Check sheet for the modelled part. Datum: model origin and axes. Units: mm. A direction names the side the tool comes from. Round coordinates to 2 decimals unless told otherwise and drop trailing zeros. Loops run counter-clockwise (first coordinate to the right, second up) from the corner with the lowest first, then second, coordinate; pieces in that order, holes last. Notation, with made-up numbers: (54.25, -10) -> (80.25, -10) arc R20 ccw to (80.25, 6) -> close; hole circle Ø8 at (13.5, 47). An arc over 180 degrees is marked (long way). One line per question, with ' | ' between items.
```python
from build123d import *

# Parameters (mm, degrees)
SKETCH_1_R          = 2.5
EXTRUDE_1_DEPTH     = 8
CHAMFER_2_SIZE      = 0.5
SKETCH_2_R          = 3.5
EXTRUDE_2_DEPTH     = 1.5
DOME_1_FACE_RADIUS  = 3.5
DOME_1_HEIGHT       = 0.8
SKETCH_3_W          = 2.012887991
SKETCH_3_H          = 3.133753739
CUT_EXTRUDE_1_DEPTH = 5


with BuildPart() as part:
    # 草图1 → 凸台-拉伸1 (new body)
    with BuildSketch(Plane.XY):
        Circle(SKETCH_1_R)
    extrude(amount=EXTRUDE_1_DEPTH)

    # 倒角2
    chamfer_2_edges = [part.edges().sort_by_distance(p)[0] for p in [
        (-2.5, 0, 8),
    ]]
    chamfer(chamfer_2_edges, length=CHAMFER_2_SIZE)

    # 草图2 → 凸台-拉伸2 (add)
    with BuildSketch(Plane(origin=(0, 0, 0), x_dir=(-1, 0, 0), z_dir=(0, 0, -1))):
        Circle(SKETCH_2_R)
    extrude(amount=EXTRUDE_2_DEPTH)

    # 圆顶1: a dome of height H over a round flat face of radius A is a cap of a sphere of radius (A * A + H * H) / (2 * H)
    dome_1_r = (DOME_1_FACE_RADIUS * DOME_1_FACE_RADIUS + DOME_1_HEIGHT * DOME_1_HEIGHT) / (2 * DOME_1_HEIGHT)
    dome_1_base = Plane((0, 0, -1.5), z_dir=(0, 0, -1))
    with Locations(dome_1_base.offset(DOME_1_HEIGHT - dome_1_r)):
        dome_1_ball = Sphere(dome_1_r, mode=Mode.PRIVATE)
    add(split(dome_1_ball, bisect_by=dome_1_base, keep=Keep.TOP, mode=Mode.PRIVATE))

    # 草图3 → 切除-拉伸1 (cut, symmetric)
    with BuildSketch(Plane(origin=(0, 0, 0), x_dir=(1, 0, 0), z_dir=(0, 1, 0))):
        with Locations((0.004540496, 2.559156118)):
            Rectangle(SKETCH_3_W, SKETCH_3_H)
    extrude(amount=CUT_EXTRUDE_1_DEPTH, both=True, mode=Mode.SUBTRACT)


solid = part.part
```
(1) Sectioned sample at B-B, the plane x = 0. Record the cut outline in (y, z), and give its area (3 significant figures).
Answer:
outline: (-3.5, -0.99) -> (3.5, -0.99) -> (3.5, 0) -> (2.5, 0) -> (2.5, 7.5) -> (2, 8) -> (-2, 8) -> (-2.5, 7.5) -> (-2.5, 0) -> (-3.5, 0) -> close | area: 46.7 mm2
(2) Sectioned sample at A-A, the plane y = 0. Record the cut outline in (x, z), and give its area (3 significant figures).
Answer:
outline: (-3.5, -1.5) arc R8.06 ccw to (-1, -2.24) -> (-1, -0.99) -> (1.01, -0.99) -> (1.01, -2.24) arc R8.06 ccw to (3.5, -1.5) -> (3.5, 0) -> (2.5, 0) -> (2.5, 7.5) -> (2, 8) -> (-2, 8) -> (-2.5, 7.5) -> (-2.5, 0) -> (-3.5, 0) -> close | area: 51.4 mm2
(3) Mould release check, pull along X, two halves, no side actions. Record for faces 1 (the face through (0, 0, 8)), 2 (the face through (-0.54, -2.44, 3.7)), 3 (the face through (1.011, 0, -1.5)): +X half, -X half, draft (parallel to the pull), parting line (faces both ways), or undercut.
Answer:
face 1: draft | face 2: parting line | face 3: undercut
(4) Set-up check for faces 4 (the face through (-2, -2, 0)), 5 (the face through (-3.233, -1.341, -0.74)), 6 (the face through (-1.002, 0, -1.5)): record each of +Z, -Z, +X, -X, +Y, -Y from which the full face is reachable in a straight line by a thin tool's end or side.
Answer:
face 4: +Z | face 5: +Z, -Z | face 6: -Z, +Y, -Y
(5) Go/stop test with flat-tipped pins: pin 1 (3 mm diameter, centred on x = -0.5, y = -0.5, fed in from -Z); pin 2 (2 mm diameter, centred on x = 2, y = -2.5, fed in from +Z); pin 3 (1 mm diameter, centred on x = 2, y = 2, fed in from +Z); pin 4 (0.6 mm diameter, centred on x = 0.5, y = -0.5, fed in from -Z). Record where each tip stops, or that it passes through.
Answer:
pin 1: stops at z = -2.24 | pin 2: stops at z = 7.8 | pin 3: stops at z = 7.67 | pin 4: stops at z = -0.99
(6) Scan lines: probe 1 along Z at (x, y) = (-0.5, -2.75); probe 2 along Z at (x, y) = (-0.25, -1); probe 3 along Y at (x, z) = (0, 1.25). Record each from-to range of solid material in increasing order.
Answer:
probe 1: z = -0.99 to 0 | probe 2: z = -0.99 to 8 | probe 3: y = -2.5 to 2.5
(7) Sectioned sample at D-D, the plane y = 3. Record the cut outline in (x, z).
Answer:
outline: (-1.8, -1.5) arc R7.48 ccw to (-1, -1.65) -> (-1, -0.99) -> (1.01, -0.99) -> (1.01, -1.65) arc R7.48 ccw to (1.8, -1.5) -> (1.8, 0) -> (-1.8, 0) -> close
(8) Sectioned sample at C-C, the plane z = 1. Record the cut outline in (x, y), and give its area (3 significant figures).
Answer:
outline: circle Ø5 at (0, 0) | area: 19.6 mm2
